Geometry check sheet. Reference: drawing and pictorial views, mm from the part's lowest x, y, z. A direction names the side the tool comes from. Give positions to 0.01 mm unless a question says otherwise; leave off trailing zeros. Order: outer loops, then holes, each group sorted by start corner. A loop starts at its lowest first (then second) coordinate and runs counter-clockwise, first axis right, second up. Notation, with made-up numbers: (57, 18.25) - (102, 18.25) arc R20 ccw to (102, 29.25) - close; hole circle Ø9 at (70.25, -6). An arc over 180 degrees is marked (long way). Answer in a Markdown table with one row per item.
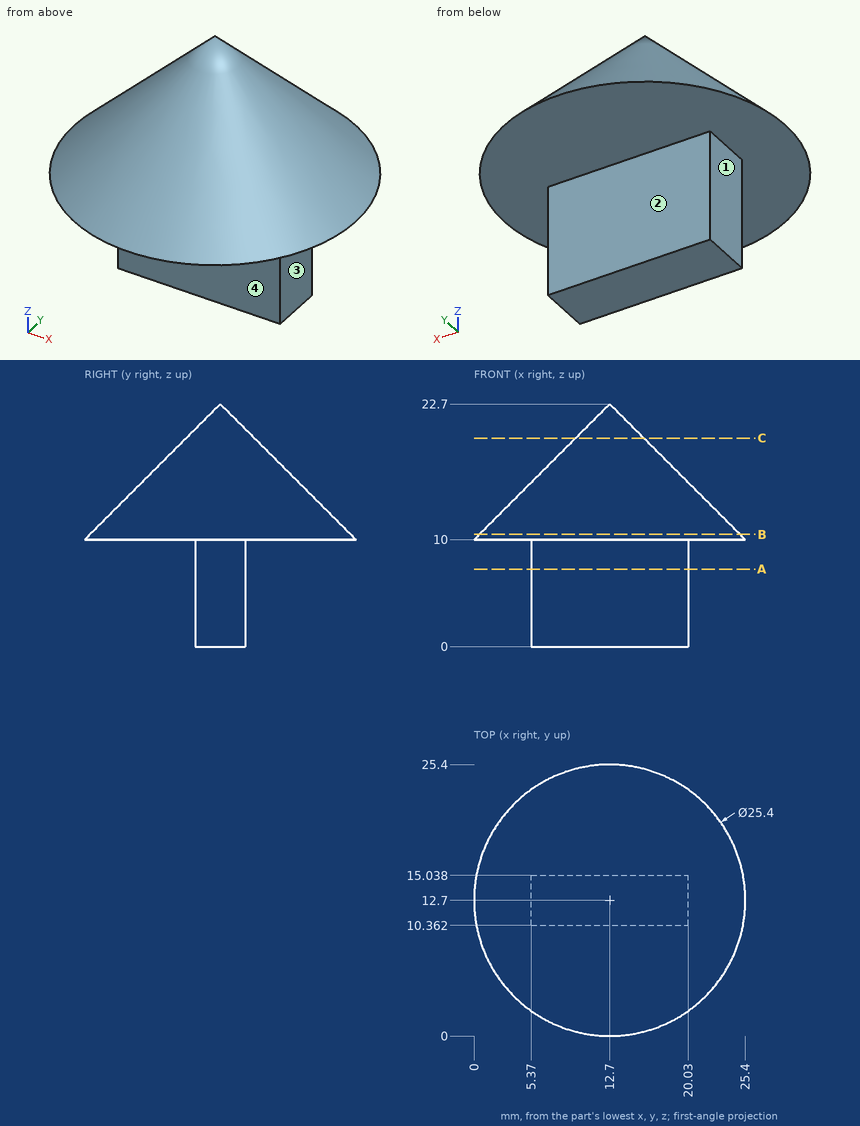
(1) Cross-section at A-A, the plane z = 7.25. Record the cut outline in (x, y).
Geometry says:
| item | result |
|---|---|
| outline | (5.37, 10.36) - (20.03, 10.36) - (20.03, 15.04) - (5.37, 15.04) - close |
(2) Gauge pin test, flat ends, axial feed: P1, Ø2.5, axis at y = 13, z = 5, coming from the -X side; P2, Ø8, axis at y = 16.5, z = 5.5, coming from the +X side; P3, Ø12, axis at x = 20.5, z = 18.5, coming from the +Y side (1 decimal). Record the tip position at first contact, or that the pin passes through.
Geometry says:
| item | result |
|---|---|
| P1 | x = 5.37 |
| P2 | x = 20.03 |
| P3 | y = 20.8 |
(3) Cross-section at C-C, the plane z = 19.5. Record the cut outline in (x, y).
Geometry says:
| item | result |
|---|---|
| outline | circle Ø6.4 at (12.7, 12.7) |
(4) Cross-section at B-B, the plane z = 10.5. Record the cut outline in (x, y), then the cut area to 3 significant figures.
Geometry says:
| item | result |
|---|---|
| outline | circle Ø24.4 at (12.7, 12.7) |
| area | 468 mm² |
(5) Thickness scan on L1, parallel to Y at x = 13.75, z = 1.75; L2, parallel to X at y = 12.5, z = 4; L3, parallel to Z at x = 19.75, y = 17. Record the ranges inside material, lowest first.
Geometry says:
| item | result |
|---|---|
| L1 | 10.36 to 15.04 |
| L2 | 5.37 to 20.03 |
| L3 | 10 to 14.44 |
(6) Access from +Z, -Z, +X, -X, +Y, -Y to the whole of each face (thin tool, end or side, straight path). Record for the marked faces 1, 2, 3 and 4.
Geometry says:
| item | result |
|---|---|
| face 1 | -Z, -X, +Y, -Y |
| face 2 | -Z, +X, -X, +Y |
| face 3 | -Z, +X, +Y, -Y |
| face 4 | -Z, +X, -X, -Y |
